Check sheet for the drawn part. Datum: minimum x, y, z corner. Units: mm. Give positions to 0.01 mm unless a question says otherwise; leave off trailing zeros. Order: outer loops, then holes, each group sorted by start corner. A loop starts at its lowest first (then second) coordinate and runs counter-clockwise, first axis right, second up.
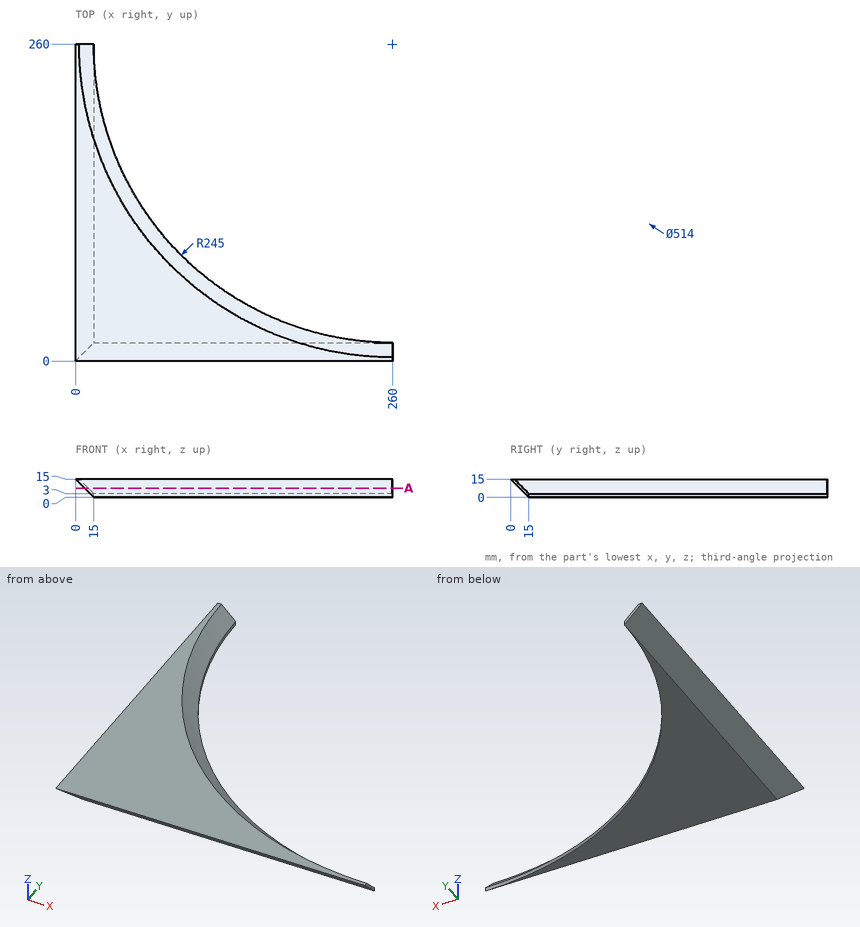
Item 1: Gauge pin test, flat ends, axial feed: pin 1 (2 mm diameter, centred on x = 223.5, z = 2, fed in from +Y); pin 2 (1.5 mm diameter, centred on x = 121.5, z = 8, fed in from -Y); pin 3 (6 mm diameter, centred on x = 194.5, z = 5, fed in from -Y). Record the tip position at first contact, or that the pin passes through.
Reported:
pin 1: stops at y = 17.89
pin 2: stops at y = 6.25
pin 3: stops at y = 7
Item 2: Sectioned sample at A-A (z = 7.5). Enter the section's corners in (x, y).
Reported:
outline: (7.5, 7.5) - (260, 7.5) - (260, 10.5) arc R249.5 cw to (10.5, 260) - (7.5, 260) - close
Item 3: Scan lines: L1, parallel to X at y = 192, z = 9.75; L2, parallel to X at y = 147, z = 12; L3, parallel to Y at x = 204, z = 11.5. Record each from-to range of solid material in increasing order.
Reported:
L1: x = 5.25 to 17.61
L2: x = 3 to 32.52
L3: y = 3.5 to 12.76
